CAD build for the part. Positions are in the model's coordinates, mm. Coordinates: 2 decimals unless noted, no trailing zeros. Loops run counter-clockwise (first coordinate to the right, second up) from the corner with the lowest first, then second, coordinate; pieces in that order, holes last. Notation, with made-up numbers: (-31, 47.25) - (0, 47.25) arc R36 cw to (0, 84.25) - close; hole circle Ø5 at (78, -26). An arc over 180 degrees is marked (long way). Put each result on its own line as item: value.
```python
from build123d import *

# Parameters (mm, degrees)
SKETCH1_R           = 19.5
BOSS_EXTRUDE1_DEPTH = 3
BOSS_EXTRUDE2_START = 37
SKETCH2_R           = 19.5
SKETCH2_R_2         = 18
BOSS_EXTRUDE2_DEPTH = 37
FILLET1_R           = 5
BOSS_EXTRUDE3_START = -6
SKETCH3_R           = 18
SKETCH3_R_2         = 17.4
BOSS_EXTRUDE3_DEPTH = 6


with BuildPart() as part:
    # Sketch1 → Boss-Extrude1 (new body)
    with BuildSketch(Plane(origin=(0, 0, 0), x_dir=(1, 0, 0), z_dir=(0, 1, 0))):
        with Locations(Location((0, 0, 0), (0, 0, 270))):
            Circle(SKETCH1_R)
    extrude(amount=BOSS_EXTRUDE1_DEPTH)

    # Sketch2 → Boss-Extrude2 (add)
    with BuildSketch(Plane(origin=(0, 0, 0), x_dir=(-1, 0, 0), z_dir=(0, -1, 0)).offset(BOSS_EXTRUDE2_START)):
        with Locations(Location((0, 0, 0), (0, 0, 90))):
            Circle(SKETCH2_R)
        with Locations(Location((0, 0, 0), (0, 0, 90))):
            Circle(SKETCH2_R_2, mode=Mode.SUBTRACT)
    extrude(amount=-BOSS_EXTRUDE2_DEPTH)

    # Fillet1
    # the kernel refuses this fillet: 5 mm, written as the material it takes off along each edge
    with BuildSketch(Plane(origin=(0, -37, 0), x_dir=(0, 0, -1), z_dir=(-1, 0, 0))) as fillet1_piece_1:
        with BuildLine():
            CenterArc((23, -3.570714214), FILLET1_R, 134.427004001, 45.572995999)
            Line((18, -3.570714214), (17.9, -3.570714214))
            Line((17.9, -3.570714214), (17.9, 0))
            Line((17.9, 0), (18, 0.1))
            ThreePointArc((18, 0.1), (18.75, 0.1), (19.43, 0.071414284))
            Line((19.43, 0.071414284), (19.5, 0))
        make_face()
    revolve(axis=Axis((0, -37, 0), (0, -1, 0)), mode=Mode.SUBTRACT)

    # Sketch3 → Boss-Extrude3 (add)
    with BuildSketch(Plane(origin=(0, 3, 0), x_dir=(1, 0, 0), z_dir=(0, 1, 0)).offset(BOSS_EXTRUDE3_START)):
        with Locations(Location((0, 0, 0), (0, 0, 270))):
            Circle(SKETCH3_R)
        with Locations(Location((0, 0, 0), (0, 0, 270))):
            Circle(SKETCH3_R_2, mode=Mode.SUBTRACT)
    extrude(amount=BOSS_EXTRUDE3_DEPTH)


solid = part.part
```
Q1. Slice it at A-A, the plane z = 0. Give the cut face in (x, y).
Determined:
outline: (-19.5, -37) arc R5 ccw to (-18, -33.43) - (-18, -3) - (-17.4, -3) - (-17.4, 0) - (17.4, 0) - (17.4, -3) - (18, -3) - (18, -33.43) arc R5 ccw to (19.5, -37) - (19.5, 3) - (-19.5, 3) - close
Q2. Slice it at C-C, the plane y = -11. Give the cut face in (x, z), then the cut area to 3 significant figures.
Determined:
outline: circle Ø39 at (0, 0); hole circle Ø36 at (0, 0)
area: 177 mm2
Q3. Wall check: L1, parallel to Z at x = 0, y = -0.85; L2, parallel to Y at x = 8.5, z = 3. Give the ranges that are in metal, low to high. Write a range as from..to.
Determined:
L1: -19.5..-17.4, 17.4..19.5
L2: 0..3
Q4. Slice it at B-B, the plane x = 0. Give the cut face in (y, z), then the cut area to 3 significant figures.
Determined:
outline: (-37, -19.5) - (3, -19.5) - (3, 19.5) - (-37, 19.5) arc R5 ccw to (-33.43, 18) - (-3, 18) - (-3, 17.4) - (0, 17.4) - (0, -17.4) - (-3, -17.4) - (-3, -18) - (-33.43, -18) arc R5 ccw to start
area: 228 mm2
Q5. Pin check, flat tips, straight feed: pin 1 Ø11 at (x, z) = (2.5, -8.5) entering from -Y; pin 2 Ø6 at (y, z) = (-21.5, 14.5) entering from +X; pin 3 Ø2 at (x, y) = (-4.5, -16.5) entering from +Z. Stop position of each tip, or through.
Determined:
pin 1: y = 0
pin 2: x = 15.75
pin 3: z = 19.18
